The listing builds one solid part. Answer for the finished solid, in the listing's coordinates (mm). A direction names the side the tool comes from. Round coordinates to 2 decimals unless told otherwise and drop trailing zeros. Loops run counter-clockwise (first coordinate to the right, second up) from the corner with the lowest first, then second, coordinate; pieces in that order, holes last. Notation, with made-up numbers: (15, 6) -> (64, 6) arc R19 ccw to (64, 10) -> close; hole circle Ø7 at (41, 78). An arc over 180 degrees is marked (long way). Answer in a Markdown table with one row per item. Add a question column.
```python
from build123d import *

# Parameters (mm, degrees)
SKETCH1_W                = 156
SKETCH1_H                = 126
BOSS_EXTRUDE1_DEPTH      = 5
CHAMFER1_SIZE            = 5
SKETCH2_R                = 1.75
CUT_EXTRUDE1_DEPTH       = 186.215391696
SKETCH3_W                = 5
SKETCH3_H                = 20
SKETCH3_W_2              = 10
SKETCH3_H_2              = 40
BOSS_EXTRUDE2_DEPTH      = 5
BOSS_EXTRUDE3_DEPTH      = 100
BOSS_EXTRUDE3_DEPTH_BACK = 10
SKETCH6_W                = 5
SKETCH6_H                = 5
SKETCH9_W                = 90
SKETCH9_H                = 28
SKETCH9_H_2              = 40
CUT_EXTRUDE3_DEPTH       = 219.48510549
FILLET1_R                = 5


with BuildPart() as part:
    # Sketch1 → Boss-Extrude1 (new body)
    with BuildSketch(Plane(origin=(0, 0, 0), x_dir=(1, 0, 0), z_dir=(0, 1, 0))):
        with Locations((78, 36.718309859)):
            Rectangle(SKETCH1_W, SKETCH1_H)
    extrude(amount=BOSS_EXTRUDE1_DEPTH)

    # Chamfer1
    chamfer1_edges = [part.edges().sort_by_distance(p)[0] for p in [
        (0, 2.5, -99.718309859),
        (156, 2.5, -99.718309859),
        (156, 2.5, 26.281690141),
        (0, 2.5, 26.281690141),
    ]]
    chamfer(chamfer1_edges, length=CHAMFER1_SIZE)

    # Sketch2 → Cut-Extrude1 (cut, through all)
    with BuildSketch(Plane(origin=(0, 5, 0), x_dir=(1, 0, 0), z_dir=(0, 1, 0))):
        with BuildLine():
            ThreePointArc((8.05, 93.418309859), (7.537436867, 94.655746726), (6.3, 95.168309859))
            Line((6.3, 95.168309859), (6.3, 93.418309859))
            Line((6.3, 93.418309859), (4.55, 93.418309859))
            ThreePointArc((4.55, 93.418309859), (6.3, 91.668309859), (8.05, 93.418309859))
        make_face()
        with BuildLine():
            Line((6.3, 93.418309859), (6.3, 95.168309859))
            ThreePointArc((6.3, 95.168309859), (5.062563133, 94.655746726), (4.55, 93.418309859))
            Line((4.55, 93.418309859), (6.3, 93.418309859))
        make_face()
        with Locations(Location((149.7, -19.981690141, 0), (0, 0, 270))):
            Circle(SKETCH2_R)
        with Locations(Location((149.7, 93.418309859, 0), (0, 0, 270))):
            Circle(SKETCH2_R)
        with Locations(Location((6.3, -19.981690141, 0), (0, 0, 90))):
            Circle(SKETCH2_R)
    extrude(amount=-CUT_EXTRUDE1_DEPTH, mode=Mode.SUBTRACT)

    # Sketch3 → Boss-Extrude2 (add)
    with BuildSketch(Plane(origin=(0, 5, 0), x_dir=(1, 0, 0), z_dir=(0, 1, 0))):
        with Locations((130.5, 46.718309859)):
            Rectangle(SKETCH3_W, SKETCH3_H)
        with Locations((125.5, 46.718309859)):
            Rectangle(SKETCH3_W, SKETCH3_H)
        Polygon((128, 36.718309859), (123, 36.718309859), (123, 16.718309859), (133, 16.718309859), (133, 36.718309859), align=None)
        with Locations((28, 36.718309859)):
            Rectangle(SKETCH3_W_2, SKETCH3_H_2)
    extrude(amount=BOSS_EXTRUDE2_DEPTH)

    # Sketch6 → Boss-Extrude3 (add, two sides: drawn at the far end of the back side and taken through both)
    with BuildSketch(Plane.ZY.offset(-123).offset(-BOSS_EXTRUDE3_DEPTH_BACK)):
        with BuildLine():
            ThreePointArc((-47.881645859, 119.68382942), (-74.400136566, 102.733481734), (-84.718309859, 73))
            Line((-84.718309859, 73), (-74.718309859, 73))
            ThreePointArc((-74.718309859, 73), (-66.480360629, 96.626686903), (-45.338292281, 110.009402901))
            Line((-45.338292281, 110.009402901), (-47.881645859, 119.68382942))
        make_face()
        with BuildLine():
            ThreePointArc((11.281690141, 73), (-6.984828126, 110.681826707), (-47.881645859, 119.68382942))
            Line((-47.881645859, 119.68382942), (-45.338292281, 110.009402901))
            ThreePointArc((-45.338292281, 110.009402901), (-13.091622957, 102.76205077), (1.281690141, 73))
            Line((1.281690141, 73), (11.281690141, 73))
        make_face()
        with BuildLine():
            Line((-26.022614728, 36.536290566), (-26.021811715, 36.53323606))
            Line((-26.021811715, 36.53323606), (-23.47926115, 26.861864046))
            ThreePointArc((-23.47926115, 26.861864046), (1.618841431, 44.116391656), (11.281690141, 73))
            Line((11.281690141, 73), (1.281690141, 73))
            ThreePointArc((1.281690141, 73), (-6.30091011, 50.223218126), (-26.022614728, 36.536290566))
        make_face()
        with BuildLine():
            ThreePointArc((-26.021811715, 36.53323606), (-33.846189614, 32.151003399), (-39.352290573, 25.072323803))
            ThreePointArc((-39.352290573, 25.072323803), (-31.340812266, 25.302174896), (-23.47926115, 26.861864046))
            Line((-23.47926115, 26.861864046), (-26.021811715, 36.53323606))
        make_face()
        with BuildLine():
            ThreePointArc((-39.352290573, 25.072323803), (-41.119015586, 20.173278405), (-41.718309859, 15))
            Line((-41.718309859, 15), (-36.718309859, 15))
            Line((-36.718309859, 15), (-31.718309859, 15))
            ThreePointArc((-31.718309859, 15), (-29.317648494, 22.124824976), (-23.47926115, 26.861864046))
            ThreePointArc((-23.47926115, 26.861864046), (-31.340812266, 25.302174896), (-39.352290573, 25.072323803))
        make_face()
        with Locations((-34.218309859, 12.5)):
            Rectangle(SKETCH6_W, SKETCH6_H)
        with Locations((-39.218309859, 12.5)):
            Rectangle(SKETCH6_W, SKETCH6_H)
    extrude(amount=BOSS_EXTRUDE3_DEPTH + BOSS_EXTRUDE3_DEPTH_BACK)

    # Sketch9 → Cut-Extrude3 (cut, through all)
    with BuildSketch(Plane(origin=(0, 5, 0), x_dir=(1, 0, 0), z_dir=(0, 1, 0))):
        with Locations((78, 70.718309859)):
            Rectangle(SKETCH9_W, SKETCH9_H)
        with Locations((78, 36.718309859)):
            Rectangle(SKETCH9_W, SKETCH9_H_2)
        with Locations((78, 2.718309859)):
            Rectangle(SKETCH9_W, SKETCH9_H)
    extrude(amount=CUT_EXTRUDE3_DEPTH, mode=Mode.SUBTRACT)

    # Fillet1
    fillet1_edges = [part.edges().sort_by_distance(p)[0] for p in [
        (28, 10, -41.718309859),
        (28, 10, -31.718309859),
        (128, 10, -31.718309859),
        (128, 10, -41.718309859),
    ]]
    fillet(fillet1_edges, radius=FILLET1_R - 0.0001)  # a hair under: the kernel refuses the full size


solid = part.part
```
Item 1: Flat-ended cylindrical pins translate along their axes: P1, Ø1.5, axis at x = 129.5, y = 8.5, coming from the -Z side; P2, Ø5, axis at x = 27.5, z = -19.5, coming from the +Y side; P3, Ø1, axis at x = 114.5, z = -71, coming from the +Y side. Find the tip coordinate at first contact, or state that the pin passes through.
Item 2: Section C-C, the plane z = -35.5 is taken. Write down the section's boundary in (x, y), and give its area (3 significant figures).
Item 3: Section B-B, the plane z = -12.5 is taken. Write down the section's boundary in (x, y), and give its area (3 significant figures).
Item 4: Section D-D, the plane y = 57 is taken. Write down the section's boundary in (x, z).
Item 5: Section A-A, the plane y = 97 is taken. Write down the section's boundary in (x, z), and give its area (3 significant figures).
Item 6: For faces 1 (the flat face through (123, 58, -1)), 2 (the flat face through (128, 10, -52)), 3 (the cylindrical face through (127.93, 11.426, -30.215)), determine the directions among +Z, -Z, +X, -X, +Y, -Y from which every point of the face is accessible in a straight line to the end or side of a thin tool.
Item 7: The mould has two halves that part along Y. Classify faces 4 (the flat face through (153.465, 2.465, -97.253)), 5 (the cylindrical face through (127.93, 11.504, -43.144)), 6 (the flat face through (77, 0, -38)), 7 (the flat face through (28, 10, -52)): +Y half, -Y half, draft (parallel to the pull), parting line (faces both ways), or undercut.
Item 8: Consider L1, parallel to Z at x = 149.7, y = 2.8; L2, parallel to Z at x = 6, y = 3; L3, parallel to X at y = 72.5, z = 11. Determine where each line is inside the solid, lowest interval first. Write a range as from..to.
Here are the results:
| question | item | result |
|---|---|---|
| 1 | P1 | stops at z = -56.72 |
| 1 | P2 | stops at y = 118.69 |
| 1 | P3 | stops at y = 5 |
| 2 | outline | (0, 0) -> (156, 0) -> (156, 5) -> (133, 5) -> (133, 30.58) -> (123, 30.58) -> (123, 5) -> (33, 5) -> (33, 30.58) -> (23, 30.58) -> (23, 5) -> (0, 5) -> close; (23, 110.98) -> (33, 110.98) -> (33, 120.98) -> (23, 120.98) -> close; (123, 110.98) -> (133, 110.98) -> (133, 120.98) -> (123, 120.98) -> close |
| 2 | area | 1,490 mm² |
| 3 | outline | (0, 0) -> (156, 0) -> (156, 5) -> (0, 5) -> close; (23, 31.56) -> (33, 31.56) -> (33, 43.72) -> (23, 43.72) -> close; (23, 102.28) -> (33, 102.28) -> (33, 114.44) -> (23, 114.44) -> close; (123, 31.56) -> (133, 31.56) -> (133, 43.72) -> (123, 43.72) -> close; (123, 102.28) -> (133, 102.28) -> (133, 114.44) -> (123, 114.44) -> close |
| 3 | area | 1,270 mm² |
| 4 | outline | (23, -2.25) -> (33, -2.25) -> (33, 8.54) -> (23, 8.54) -> close; (123, -2.25) -> (133, -2.25) -> (133, 8.54) -> (123, 8.54) -> close |
| 5 | outline | (23, -78.29) -> (33, -78.29) -> (33, -66.18) -> (23, -66.18) -> close; (23, -7.26) -> (33, -7.26) -> (33, 4.85) -> (23, 4.85) -> close; (123, -78.29) -> (133, -78.29) -> (133, -66.18) -> (123, -66.18) -> close; (123, -7.26) -> (133, -7.26) -> (133, 4.85) -> (123, 4.85) -> close |
| 5 | area | 484 mm² |
| 6 | face 1 | +Z, -Z, +Y |
| 6 | face 2 | -Z, +X, -X |
| 6 | face 3 | +Z, +X, -X |
| 7 | face 4 | draft |
| 7 | face 5 | undercut |
| 7 | face 6 | -Y half |
| 7 | face 7 | undercut |
| 8 | L1 | z = -99.72..-95.17, -91.67..18.23, 21.73..26.28 |
| 8 | L2 | z = -99.72..-95.14, -91.69..18.26, 21.71..26.28 |
| 8 | L3 | x = 23..33, 123..133 |
